Autodesk Inventor part; units mm, degrees
ref_plane "YZ Plane" through (0, 0, 0) normal (1, 0, 0) x (0, 1, 0)
ref_plane "XZ Plane" through (0, 0, 0) normal (0, 1, 0) x (-1, 0, 0)
ref_plane "XY Plane" through (0, 0, 0) normal (0, 0, 1) x (1, 0, 0)
sketch "Sketch1" plane through (0, 0, 0) normal (1, 0, 0) x (0, 1, 0)
  circle A0 centre (0, 0) radius 145
  circle A1 centre (0, 0) radius 115
  circle A2 centre (0, 0) radius 130
  circle A3 centre (130, 0) radius 8
  circle A4 centre (40.1722, 123.6373) radius 8
  circle A5 centre (-105.1722, 76.4121) radius 8
  circle A6 centre (-105.1722, -76.4121) radius 8
  circle A7 centre (40.1722, -123.6373) radius 8
  dimension "d2" = 260
  dimension "d0" = 290
  dimension "d1" = 230
  dimension "d3" = 16
  dimension "d26" = 360
extrude "Extrusion1" add sketch "Sketch1" along normal blind 10 contours A0 | A3 A2 A7 A6 A5 A4
sketch "Sketch2" plane through (0, 0, 0) normal (0, 0, 1) x (1, 0, 0)
  line L0 (0, -145) -> (0, 145)
  line L1 (0, 115) -> (0, 115.4469)
  line L2 (0, 115.4469) -> (0, 105.4469)
  line L3 (10, -145) -> (10, 145)
  line L4 (10, 120.4469) -> (10, 95.4469)
  line L5 (-2, 0) -> (12, 0)
  line L6 (0, 105.4469) -> (0, 115)
  line L7 (10, 115) -> (10, -115)
  line L8 (10, 115) -> (0, 115)
  line L9 (10, 115) -> (10, 95.4469)
  line L10 (0, 95.4469) -> (0, 105.4469)
  line L11 (0, 95.4469) -> (10, 95.4469)
  point P0 (0, 0)
revolve "Revolution1" add sketch "Sketch2" angle 360 about axis through (-10, 0, 0) along (1, 0, 0) contours L0 L8 L3 L11
sketch "Sketch3" plane through (0, 0, 0) normal (0, 0, 1) x (1, 0, 0)
  line L0 (15, 90.4469) -> (25, 90.4469)
  line L1 (25, 90.4469) -> (25, 84.4469)
  line L2 (25, 84.4469) -> (15, 84.4469)
  line L3 (10.0111, 105.4469) -> (0, 105.4469)
  line L4 (0, 105.4469) -> (0, 84.4469)
  line L5 (10.0111, 105.4469) -> (0, 105.4469)
  line L6 (15, 84.4469) -> (15, 80.4469)
  line L7 (15, 80.4469) -> (25, 80.4469)
  line L8 (25, 80.4469) -> (25, 75.4469)
  line L9 (25, 75.4469) -> (25, 74.4469)
  line L10 (25, 74.4469) -> (15, 74.4469)
  line L11 (15, 74.4469) -> (15, 70.4469)
  line L12 (15, 70.4469) -> (25, 70.4469)
  line L13 (25, 70.4469) -> (25, 64.4469)
  line L14 (25, 64.4469) -> (0, 64.4469)
  line L15 (0, 64.4469) -> (0, 84.4469)
  line L16 (10.0111, 105.4469) -> (10.0111, 90.4469)
  line L17 (10.0111, 90.4469) -> (15, 90.4469)
  line L18 (-5, 0) -> (30, 0)
  point P0 (0, 0)
revolve "Revolution2" add sketch "Sketch3" angle 360 about axis through (-10, 0, 0) along (1, 0, 0)
thread "Thread7"
thread "Thread8"
thread "Thread9"
thread "Thread10"
thread "Thread11"
properties part number "LABYRINTHOSeisodos"
Design review of the part built by this model. Coordinates are the model's own, in mm. A direction names the side the tool comes from. Coordinates: 2 decimals unless noted, no trailing zeros. Loops run counter-clockwise (first coordinate to the right, second up) from the corner with the lowest first, then second, coordinate; pieces in that order, holes last.
Item 1: Draft analysis for pull direction Y (two halves, no side actions). For faces 3 (the flat face through (10.011, 46, 79)), 4 (the cylindrical face through (19.93, -59.08, 45.3)), 5 (the cylindrical face through (4.93, 137.39, 3.06)), 6 (the cylindrical face through (4.93, 138.304, -43.554)), state which applies: pulls with the +Y half, pulls with the -Y half, needs draft (parallel to the pull), parting line crosses it, or undercut.
Completed:
face 3: needs draft
face 4: undercut
face 5: undercut
face 6: parting line crosses it
Item 2: Add section A-A (x = 18.5). Write out the cut boundary in (y, z), and give its area (3 significant figures).
Completed:
outline: circle Ø180.89 at (0, 0); circle Ø160.89 at (0, 0); circle Ø140.89 at (0, 0); hole circle Ø168.89 at (0, 0); hole circle Ø148.89 at (0, 0); hole circle Ø128.89 at (0, 0)
area: 8,760 mm2
Item 3: Add section D-D (z = 0). Give the number of separate pieces and of enclosed holes in the cut face, and give its area (3 significant figures).
Completed:
separate pieces: 3
enclosed holes: 0
area: 2,070 mm2
Item 4: Wall thickness on L1, parallel to Z at x = 19, y = 0; L2, parallel to Z at x = 22.25, y = -36; L3, parallel to X at y = 7.5, z = -96.5: over which ranges is each line inside the solid? List them lowest first.
Completed:
L1: z = -90.45 to -84.45, -80.45 to -74.45, -70.45 to -64.45, 64.45 to 70.45, 74.45 to 80.45, 84.45 to 90.45
L2: z = -82.97 to -76.39, -71.94 to -65.16, -60.55 to -53.45, 53.45 to 60.55, 65.16 to 71.94, 76.39 to 82.97
L3: x = 0 to 10.01
Item 5: Clearance check with flat-ended pins moving along their axes: pin 1 (3 mm diameter, centred on x = 5.5, z = 23.5, fed in from +Y); pin 2 (21 mm diameter, centred on y = -105.17, z = 76.41, fed in from +X); pin 3 (5 mm diameter, centred on x = 15, z = 61, fed in from +Y). State where each tip first meets the part, or that it passes through.
Completed:
pin 1: stops at y = 143.32
pin 2: stops at x = 10
pin 3: stops at y = 68.98
Item 6: For faces 1 (the cylindrical face through (20.07, 67.194, 21.16)), 2 (the cylindrical face through (4.93, 39.131, 115.705)), list the 3-axis set-ups (+Z, -Z, +X, -X, +Y, -Y) from which the entire face can be reached by the end or side of a thin tool; tool diameter is ignored.
Completed:
face 1: +X
face 2: +X, -X
